Design review of the part shown in the three views and the two pictorial views. Dimensions are in mm from the part's minimum x, y and z. Round coordinates to 2 decimals unless told otherwise and drop trailing zeros. Order: outer loops, then holes, each group sorted by start corner. A loop starts at its lowest first (then second) coordinate and runs counter-clockwise, first axis right, second up. Notation, with made-up numbers: M 61.25,-12 L 72.25,-12 A35 cw 72.25,26 Z; hole C 11,1.25 d3. An arc over 180 degrees is marked long. Write each question's results on one line, items separated by ' | '. Start each with the question number.
Item 1: Wall thickness on line 1 (Z direction, x = 14.25, y = 1.65); line 2 (Z direction, x = 25, y = 1.65); line 3 (X direction, y = 1, z = 22): over which ranges is each line inside the solid? List them lowest first. Write a range as [from, to].
Item 2: Take a section at A-A, the plane z = 22. Write out the cut boundary in (x, y).
Item 3: Take a section at B-B, the plane z = 39.6. Write out the cut boundary in (x, y), plus the area to 3 significant figures.
Item 4: Take a section at C-C, the plane y = 1. Count the separate pieces of the cut face and the enclosed holes in it, plus the area to 3 significant figures.
Item 5: Clearance check with flat-ended pins moving along their axes: pin 1 (1.5 mm diameter, centred on x = 7.5, y = 1, fed in from +Z); pin 2 (1.5 mm diameter, centred on y = 1.5, z = 48.5, fed in from +X); pin 3 (0.9 mm diameter, centred on y = 1.5, z = 45.5, fed in from +X). State where each tip first meets the part, or that it passes through.
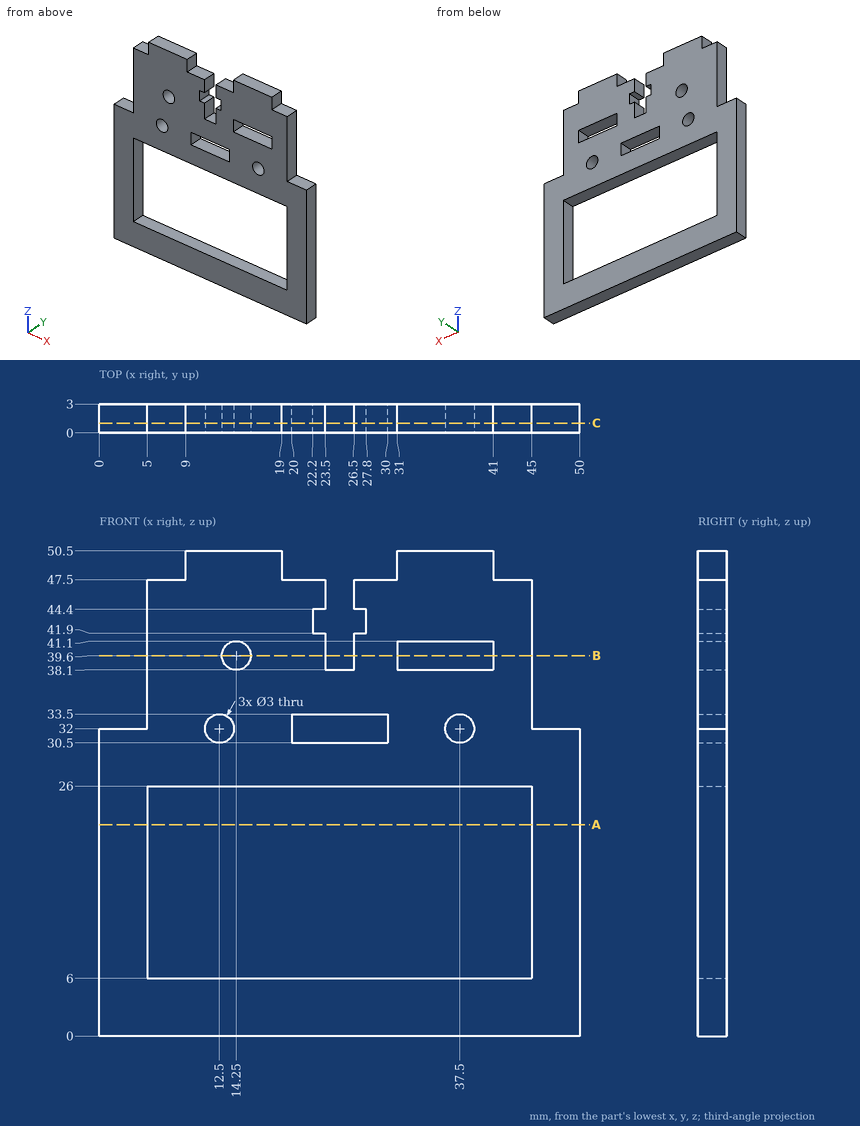
Results list:
1) line 1: [0, 6], [26, 38.1], [41.1, 50.5] | line 2: [0, 6], [26, 30.5], [33.5, 38.1] | line 3: [0, 5], [45, 50]
2) outline: M 0,0 L 5,0 L 5,3 L 0,3 Z; M 45,0 L 50,0 L 50,3 L 45,3 Z
3) outline: M 5,0 L 12.75,0 L 12.75,3 L 5,3 Z; M 15.75,0 L 23.5,0 L 23.5,3 L 15.75,3 Z; M 26.5,0 L 31,0 L 31,3 L 26.5,3 Z; M 41,0 L 45,0 L 45,3 L 41,3 Z | area: 72.0 mm²
4) separate pieces: 1 | enclosed holes: 6 | area: 1,360 mm²
5) pin 1: z = 47.5 | pin 2: x = 41 | pin 3: x = 45
